from build123d import *

# Parameters (mm, degrees)
F2_R     = 2.032
F3_DEPTH = 15.875
F4_DEPTH = 10.9982


# Not quite as in the source:
# - a feature names something its author has since deleted; it is built from what else it names


with BuildPart() as f1:
    # F0 (on Top) → F1 (revolve)
    with BuildSketch(Plane.XY):
        with BuildLine():
            Line((0, -5.1666409709), (0, -12.1516409709))
            Line((0, -12.1516409709), (45.72, -12.1516409709))
            ThreePointArc((45.72, -12.1516409709), (42.9147529825, -8.6591409709), (45.72, -5.1666409709))
            Line((45.72, -5.1666409709), (0, -5.1666409709))
        make_face()
    revolve(axis=Axis((0, -8.561744864, 0), (0, 1, 0)))

    # F2 (on Front) → F3 (cut)
    with BuildSketch(Plane.XZ):
        with BuildLine():
            Line((13.97, 3.6661742094), (13.97, -3.6661742094))
            Line((13.97, -3.6661742094), (38.6802071591, -16.0932599922))
            ThreePointArc((38.6802071591, -16.0932599922), (41.8782799617, 1.5705660984), (37.3345500424, 18.9369975174))
            Line((37.3345500424, 18.9369975174), (13.97, 3.6661742094))
        make_face()
        with BuildLine():
            Line((3.81, 41.7094333604), (3.81, 13.9314619955))
            Line((3.81, 13.9314619955), (10.16, 10.2652877862))
            Line((10.16, 10.2652877862), (34.2119266748, 24.1516741264))
            ThreePointArc((34.2119266748, 24.1516741264), (20.9542761873, 36.2954737188), (3.81, 41.7094333604))
        make_face()
        with BuildLine():
            Line((-34.2388233597, 24.0958361272), (-10.16, 10.2652877862))
            Line((-10.16, 10.2652877862), (-3.81, 13.9314619955))
            Line((-3.81, 13.9314619955), (-3.81, 41.7173788368))
            ThreePointArc((-3.81, 41.7173788368), (-20.9781685322, 36.2803485402), (-34.2388233597, 24.0958361272))
        make_face()
        with BuildLine():
            Line((-38.6893950171, -16.0623838358), (-13.97, -3.6661742094))
            Line((-13.97, -3.6661742094), (-13.97, 3.6661742094))
            Line((-13.97, 3.6661742094), (-37.3405062231, 18.9372899969))
            ThreePointArc((-37.3405062231, 18.9372899969), (-41.8787701809, 1.5863648371), (-38.6893950171, -16.0623838358))
        make_face()
        with BuildLine():
            Line((-3.81, -13.9314619955), (-10.16, -10.2652877862))
            Line((-10.16, -10.2652877862), (-34.3038742814, -23.844345572))
            ThreePointArc((-34.3038742814, -23.844345572), (-20.4303998238, -36.5921428083), (-2.2874128339, -41.6726596109))
            Line((-2.2874128339, -41.6726596109), (-3.81, -13.9314619955))
        make_face()
        with BuildLine():
            Line((10.16, -10.2652877862), (3.81, -13.9314619955))
            Line((3.81, -13.9314619955), (5.4400267393, -41.5192010913))
            ThreePointArc((5.4400267393, -41.5192010913), (22.3730839146, -35.4381883413), (35.1536490306, -22.7746857971))
            Line((35.1536490306, -22.7746857971), (10.16, -10.2652877862))
        make_face()
        Circle(F2_R)
    extrude(amount=F3_DEPTH, mode=Mode.SUBTRACT)

    # F2 (on Front) → F4 (cut)
    with BuildSketch(Plane.XZ):
        Polygon((-7.0386894402, 0.071686571), (-3.5814271117, -6.059840579), (3.4572623285, -6.1315271501), (7.0386894402, -0.071686571), (3.5814271117, 6.059840579), (-3.4572623285, 6.1315271501), align=None)
        Circle(F2_R, mode=Mode.SUBTRACT)
    extrude(amount=F4_DEPTH, mode=Mode.SUBTRACT)


solid = f1.part
Here's how the part is built. I have some questions about the finished solid (model axes, mm). A direction names the side the tool comes from. Round coordinates to 2 decimals unless told otherwise and drop trailing zeros. Write each loop counter-clockwise with the first axis right and the second up, starting at its lowest first coordinate (ties: lowest second). Pieces come first, ordered by that corner, then holes.
1. I need wall thicknesses on L1, parallel to X at y = -11.3, z = 0; L2, parallel to Z at x = -4.5, y = -6; L3, parallel to Z at x = 16.5, y = -11. Which ranges of each line are inside material? Lowest first, please.
2. For faces 1 (the flat face through (5.223, -8.042, -3.144)), 2 (the cylindrical face through (-41.87, -8.61, 1.84)), which set-ups out of +Z, -Z, +X, -X, +Y, -Y let a thin tool reach every point of the face, with its end or its side?
3. Suppose I cut it at B-B (x = 0). List the corners of the cut face in (y, z) for me, and give its area (3 significant figures).
4. Will these pins go through, and if not, where does the flat tip stop? pin 1 Ø2 at (y, z) = (-9.5, 31.5) entering from +X; pin 2 Ø10 at (x, z) = (14.5, 15) entering from -Y; pin 3 Ø2 at (y, z) = (-7.5, 31.5) entering from -X; pin 4 Ø6.5 at (x, z) = (0, 0) entering from +Y.
5. Suppose I cut it at A-A (y = -8). State how many separate pieces and enclosed holes the cut face has, and give its area (3 significant figures).
Answer sheet:
1. L1: x = -44.08 to -41.91, -13.97 to -2.03, 2.03 to 13.97, 41.91 to 44.08
1. L2: z = -43.87 to -41.53, -13.53 to -4.43, 4.37 to 13.53, 41.65 to 43.87
1. L3: z = -40.56 to -38.52, -13.44 to -4.94, 5.32 to 13.93, 38.52 to 40.56
2. face 1: +Y
2. face 2: +Y, -Y
3. outline: (-12.15, -45.72) arc R3.58 cw to (-5.17, -45.72) - (-5.17, -6.1) - (-11, -6.1) - (-11, -2.03) - (-12.15, -2.03) - close; (-12.15, 2.03) - (-11, 2.03) - (-11, 6.1) - (-5.17, 6.1) - (-5.17, 45.72) arc R3.58 cw to (-12.15, 45.72) - close
3. area: 534 mm2
4. pin 1: stops at x = 30.43
4. pin 2: stops at y = -12.15
4. pin 3: stops at x = -30.65
4. pin 4: stops at y = -11
5. separate pieces: 1
5. enclosed holes: 7
5. area: 2,040 mm2
